from build123d import *

# Parameters (mm, degrees)
CROQUIS1_W              = 40
CROQUIS1_H              = 19
SALIENTE_EXTRUIR1_DEPTH = 36
SALIENTE_EXTRUIR2_DEPTH = 2.5
REDONDEO1_R             = 0.5
REDONDEO2_R             = 0.5
SALIENTE_EXTRUIR3_DEPTH = 2
SALIENTE_EXTRUIR4_DEPTH = 2
CROQUIS5_R              = 6.5
SALIENTE_EXTRUIR5_DEPTH = 1
CROQUIS6_R              = 5
SALIENTE_EXTRUIR6_DEPTH = 0.5
CROQUIS7_R              = 3
SALIENTE_EXTRUIR7_DEPTH = 5
SALIENTE_EXTRUIR8_START = -4
CROQUIS8_R              = 3
SALIENTE_EXTRUIR8_DEPTH = 4
CROQUIS9_R              = 2
CORTAR_EXTRUIR1_DEPTH   = 5
CHAFL_N1_SIZE           = 0.25
SALIENTE_EXTRUIR9_DEPTH = 1.75


with BuildPart() as part:
    # Croquis1 → Saliente-Extruir1 (new body)
    with BuildSketch(Plane(origin=(0, 0, 0), x_dir=(1, 0, 0), z_dir=(0, 1, 0))):
        with Locations((20, -9.5)):
            Rectangle(CROQUIS1_W, CROQUIS1_H)
    extrude(amount=SALIENTE_EXTRUIR1_DEPTH)

    # Croquis2 → Saliente-Extruir2 (add)
    with BuildSketch(Plane(origin=(0, 31, 0), x_dir=(-1, 0, 0), z_dir=(0, 1, 0))):
        with BuildLine():
            ThreePointArc((-46.515564437, 3.5), (-42.25, 4.5), (-46.515564437, 5.5))
            Line((-46.515564437, 5.5), (-47.5, 5.5))
            Line((-47.5, 5.5), (-47.5, 13.5))
            Line((-47.5, 13.5), (-46.515564437, 13.5))
            ThreePointArc((-46.515564437, 13.5), (-42.25, 14.5), (-46.515564437, 15.5))
            Line((-46.515564437, 15.5), (-47.5, 15.5))
            Line((-47.5, 15.5), (-47.5, 18.25))
            Line((-47.5, 18.25), (-40, 18.25))
            Line((-40, 18.25), (-40, 0.75))
            Line((-40, 0.75), (-47.5, 0.75))
            Line((-47.5, 0.75), (-47.5, 3.5))
            Line((-47.5, 3.5), (-46.515564437, 3.5))
        make_face()
        with BuildLine():
            Line((6.515564437, 13.5), (7.5, 13.5))
            Line((7.5, 13.5), (7.5, 5.5))
            Line((7.5, 5.5), (6.515564437, 5.5))
            ThreePointArc((6.515564437, 5.5), (2.25, 4.5), (6.515564437, 3.5))
            Line((6.515564437, 3.5), (7.5, 3.5))
            Line((7.5, 3.5), (7.5, 0.75))
            Line((7.5, 0.75), (0, 0.75))
            Line((0, 0.75), (0, 18.25))
            Line((0, 18.25), (7.5, 18.25))
            Line((7.5, 18.25), (7.5, 15.5))
            Line((7.5, 15.5), (6.515564437, 15.5))
            ThreePointArc((6.515564437, 15.5), (2.25, 14.5), (6.515564437, 13.5))
        make_face()
    extrude(amount=-SALIENTE_EXTRUIR2_DEPTH)

    # Redondeo1
    redondeo1_edges = [part.edges().sort_by_distance(p)[0] for p in [
        (0, 18, 0),
        (40, 18, 0),
        (40, 18, 19),
        (0, 18, 19),
    ]]
    fillet(redondeo1_edges, radius=REDONDEO1_R)

    # Redondeo2
    redondeo2_edges = [part.edges().sort_by_distance(p)[0] for p in [
        (0, 36, 9.5),
        (20, 36, 0),
        (20, 36, 19),
        (40, 36, 9.5),
        (39.853553391, 36, 18.853553391),
        (39.853553391, 36, 0.146446609),
        (0.146446609, 36, 18.853553391),
        (0.146446609, 36, 0.146446609),
    ]]
    fillet(redondeo2_edges, radius=REDONDEO2_R)

    # Croquis3 → Saliente-Extruir3 (add)
    with BuildSketch(Plane(origin=(0, 36, 0), x_dir=(1, 0, 0), z_dir=(0, 1, 0))):
        with BuildLine():
            Line((34.5, -18.25), (34.5, -0.75))
            Line((34.5, -0.75), (14.5, -0.75))
            Line((14.5, -0.75), (13.699662147, -0.75))
            ThreePointArc((13.699662147, -0.75), (17.918231823, -4.25103774), (19.5, -9.5))
            ThreePointArc((19.5, -9.5), (17.918231823, -14.74896226), (13.699662147, -18.25))
            Line((13.699662147, -18.25), (14.5, -18.25))
            Line((14.5, -18.25), (34.5, -18.25))
        make_face()
    extrude(amount=SALIENTE_EXTRUIR3_DEPTH)

    # Croquis4 → Saliente-Extruir4 (add, symmetric)
    with BuildSketch(Plane(origin=(0, 36, 0), x_dir=(1, 0, 0), z_dir=(0, 1, 0))):
        with BuildLine():
            ThreePointArc((19.5, -9.5), (17.918231823, -4.25103774), (13.699662147, -0.75))
            ThreePointArc((13.699662147, -0.75), (13.3728388, -0.618898805), (13.041381265, -0.5))
            Line((13.041381265, -0.5), (6.958618735, -0.5))
            ThreePointArc((6.958618735, -0.5), (0.5, -9.5), (6.958618735, -18.5))
            Line((6.958618735, -18.5), (13.041381265, -18.5))
            ThreePointArc((13.041381265, -18.5), (13.3728388, -18.381101195), (13.699662147, -18.25))
            ThreePointArc((13.699662147, -18.25), (17.918231823, -14.74896226), (19.5, -9.5))
        make_face()
        with BuildLine():
            ThreePointArc((6.958618735, -18.5), (10, -19), (13.041381265, -18.5))
            Line((13.041381265, -18.5), (6.958618735, -18.5))
        make_face()
        with BuildLine():
            Line((6.958618735, -0.5), (13.041381265, -0.5))
            ThreePointArc((13.041381265, -0.5), (10, 0), (6.958618735, -0.5))
        make_face()
    extrude(amount=SALIENTE_EXTRUIR4_DEPTH, both=True)

    # Croquis5 → Saliente-Extruir5 (add)
    with BuildSketch(Plane(origin=(0, 38, 0), x_dir=(1, 0, 0), z_dir=(0, 1, 0))):
        with Locations(Location((10, -9.5, 0), (0, 0, 270))):
            Circle(CROQUIS5_R)
    extrude(amount=SALIENTE_EXTRUIR5_DEPTH)

    # Croquis6 → Saliente-Extruir6 (add)
    with BuildSketch(Plane(origin=(0, 39, 0), x_dir=(1, 0, 0), z_dir=(0, 1, 0))):
        with Locations(Location((10, -9.5, 0), (0, 0, 270))):
            Circle(CROQUIS6_R)
    extrude(amount=SALIENTE_EXTRUIR6_DEPTH)

    # Croquis7 → Saliente-Extruir7 (add)
    with BuildSketch(Plane(origin=(0, 39.5, 0), x_dir=(1, 0, 0), z_dir=(0, 1, 0))):
        with Locations(Location((10, -9.5, 0), (0, 0, 270))):
            Circle(CROQUIS7_R)
    extrude(amount=SALIENTE_EXTRUIR7_DEPTH)

    # Croquis8 → Saliente-Extruir8 (add)
    with BuildSketch(Plane(origin=(0, 44.5, 0), x_dir=(1, 0, 0), z_dir=(0, 1, 0)).offset(SALIENTE_EXTRUIR8_START)):
        with Locations(Location((10, -9.5, 0), (0, 0, 270))):
            Circle(CROQUIS8_R)
        with BuildLine():
            ThreePointArc((8.5, -6.901923789), (8.11283957, -7.040604645), (7.878679656, -7.378679656))
            ThreePointArc((7.878679656, -7.378679656), (8.173715713, -7.119939979), (8.5, -6.901923789))
        make_face()
        with BuildLine():
            ThreePointArc((9.223542865, -6.602222521), (8.81368136, -6.635973449), (8.5, -6.901923789))
            ThreePointArc((8.5, -6.901923789), (8.851949703, -6.728361402), (9.223542865, -6.602222521))
        make_face()
        with BuildLine():
            ThreePointArc((10, -6.5), (9.595368804, -6.42652093), (9.223542865, -6.602222521))
            ThreePointArc((9.223542865, -6.602222521), (9.608421423, -6.525665416), (10, -6.5))
        make_face()
        with BuildLine():
            ThreePointArc((10.776457135, -6.602222521), (10.404631196, -6.42652093), (10, -6.5))
            ThreePointArc((10, -6.5), (10.391578577, -6.525665416), (10.776457135, -6.602222521))
        make_face()
        with BuildLine():
            ThreePointArc((11.5, -6.901923789), (11.18631864, -6.635973449), (10.776457135, -6.602222521))
            ThreePointArc((10.776457135, -6.602222521), (11.148050297, -6.728361402), (11.5, -6.901923789))
        make_face()
        with BuildLine():
            ThreePointArc((12.121320344, -7.378679656), (11.88716043, -7.040604645), (11.5, -6.901923789))
            ThreePointArc((11.5, -6.901923789), (11.826284287, -7.119939979), (12.121320344, -7.378679656))
        make_face()
        with BuildLine():
            ThreePointArc((12.598076211, -8), (12.771638598, -8.351949703), (12.897777479, -8.723542865))
            ThreePointArc((12.897777479, -8.723542865), (12.864026551, -8.31368136), (12.598076211, -8))
        make_face()
        with BuildLine():
            ThreePointArc((12.897777479, -8.723542865), (12.974334584, -9.108421423), (13, -9.5))
            ThreePointArc((13, -9.5), (13.07347907, -9.095368804), (12.897777479, -8.723542865))
        make_face()
        with BuildLine():
            ThreePointArc((12.121320344, -7.378679656), (12.380060021, -7.673715713), (12.598076211, -8))
            ThreePointArc((12.598076211, -8), (12.459395355, -7.61283957), (12.121320344, -7.378679656))
        make_face()
        with BuildLine():
            ThreePointArc((7.878679656, -7.378679656), (7.540604645, -7.61283957), (7.401923789, -8))
            ThreePointArc((7.401923789, -8), (7.619939979, -7.673715713), (7.878679656, -7.378679656))
        make_face()
        with BuildLine():
            ThreePointArc((7.401923789, -11), (7.440963384, -11.204433973), (7.540604645, -11.38716043))
            ThreePointArc((7.540604645, -11.38716043), (7.691315793, -11.530699585), (7.878679656, -11.621320344))
            ThreePointArc((7.878679656, -11.621320344), (7.619939979, -11.326284287), (7.401923789, -11))
        make_face()
        with BuildLine():
            ThreePointArc((7.102222521, -10.276457135), (7.135973449, -10.68631864), (7.401923789, -11))
            ThreePointArc((7.401923789, -11), (7.228361402, -10.648050297), (7.102222521, -10.276457135))
        make_face()
        with BuildLine():
            ThreePointArc((7, -9.5), (6.92652093, -9.904631196), (7.102222521, -10.276457135))
            ThreePointArc((7.102222521, -10.276457135), (7.025665416, -9.891578577), (7, -9.5))
        make_face()
        with BuildLine():
            ThreePointArc((7.102222521, -8.723542865), (6.92652093, -9.095368804), (7, -9.5))
            ThreePointArc((7, -9.5), (7.025665416, -9.108421423), (7.102222521, -8.723542865))
        make_face()
        with BuildLine():
            ThreePointArc((7.401923789, -8), (7.135973449, -8.31368136), (7.102222521, -8.723542865))
            ThreePointArc((7.102222521, -8.723542865), (7.228361402, -8.351949703), (7.401923789, -8))
        make_face()
        with BuildLine():
            ThreePointArc((7.878679656, -11.621320344), (7.969300415, -11.808684207), (8.11283957, -11.959395355))
            ThreePointArc((8.11283957, -11.959395355), (8.295566027, -12.059036616), (8.5, -12.098076211))
            ThreePointArc((8.5, -12.098076211), (8.173715713, -11.880060021), (7.878679656, -11.621320344))
        make_face()
        with BuildLine():
            ThreePointArc((9.223542865, -12.397777479), (8.851949703, -12.271638598), (8.5, -12.098076211))
            ThreePointArc((8.5, -12.098076211), (8.81368136, -12.364026551), (9.223542865, -12.397777479))
        make_face()
        with BuildLine():
            ThreePointArc((10, -12.5), (9.608421423, -12.474334584), (9.223542865, -12.397777479))
            ThreePointArc((9.223542865, -12.397777479), (9.595368804, -12.57347907), (10, -12.5))
        make_face()
        with BuildLine():
            ThreePointArc((10.776457135, -12.397777479), (10.391578577, -12.474334584), (10, -12.5))
            ThreePointArc((10, -12.5), (10.404631196, -12.57347907), (10.776457135, -12.397777479))
        make_face()
        with BuildLine():
            ThreePointArc((11.5, -12.098076211), (11.148050297, -12.271638598), (10.776457135, -12.397777479))
            ThreePointArc((10.776457135, -12.397777479), (11.18631864, -12.364026551), (11.5, -12.098076211))
        make_face()
        with BuildLine():
            ThreePointArc((12.121320344, -11.621320344), (11.826284287, -11.880060021), (11.5, -12.098076211))
            ThreePointArc((11.5, -12.098076211), (11.88716043, -11.959395355), (12.121320344, -11.621320344))
        make_face()
        with BuildLine():
            ThreePointArc((12.598076211, -11), (12.380060021, -11.326284287), (12.121320344, -11.621320344))
            ThreePointArc((12.121320344, -11.621320344), (12.459395355, -11.38716043), (12.598076211, -11))
        make_face()
        with BuildLine():
            ThreePointArc((12.897777479, -10.276457135), (12.771638598, -10.648050297), (12.598076211, -11))
            ThreePointArc((12.598076211, -11), (12.864026551, -10.68631864), (12.897777479, -10.276457135))
        make_face()
        with BuildLine():
            ThreePointArc((13, -9.5), (12.974334584, -9.891578577), (12.897777479, -10.276457135))
            ThreePointArc((12.897777479, -10.276457135), (13.07347907, -9.904631196), (13, -9.5))
        make_face()
    extrude(amount=SALIENTE_EXTRUIR8_DEPTH)

    # Croquis9 → Cortar-Extruir1 (cut)
    with BuildSketch(Plane(origin=(0, 44.5, 0), x_dir=(1, 0, 0), z_dir=(0, 1, 0))):
        with Locations(Location((10, -9.5, 0), (0, 0, 270))):
            Circle(CROQUIS9_R)
    extrude(amount=-CORTAR_EXTRUIR1_DEPTH, mode=Mode.SUBTRACT)

    # Chaflán1
    chafl_n1_edges = [part.edges().sort_by_distance(p)[0] for p in [
        (10, 44.5, 7.5),
    ]]
    chamfer(chafl_n1_edges, length=CHAFL_N1_SIZE)

    # Croquis10 → Saliente-Extruir9 (add)
    with BuildSketch(Plane(origin=(0, 36, 0), x_dir=(1, 0, 0), z_dir=(0, 1, 0))):
        with BuildLine():
            ThreePointArc((34.5, -14), (36, -9.5), (34.5, -5))
            Line((34.5, -5), (34.5, -14))
        make_face()
    extrude(amount=SALIENTE_EXTRUIR9_DEPTH)


solid = part.part
For this review, take the finished solid that the model builds, in its own axes (mm). A direction names the side the tool comes from. Give positions to 0.01 mm unless a question says otherwise; leave off trailing zeros. Loops run counter-clockwise (first coordinate to the right, second up) from the corner with the lowest first, then second, coordinate; pieces in that order, holes last. Notation, with made-up numbers: M -20.75,15.5 L 29.25,15.5 A15 cw 29.25,26.5 Z; hole C 4.5,-14.5 d11. An arc over 180 degrees is marked long. Put each result on its own line as item: value. Start each with the question number.
(1) Machinability: for faces 5 (the flat face through (10, 39.5, 9)), 6 (the flat face through (-3, 31, 10)), 7 (the flat face through (44, 30, 0.75)), which of the approach directions +Z, -Z, +X, -X, +Y, -Y give a long, thin tool a straight path to every point of the face, cutting with its end or side? Answer none if there is none.
(2) Add section C-C, the plane x = 33.5. Write out the cut boundary in (y, z), then the cut area to 3 significant figures.
(3) The part is to be moulded in two halves that separate along Z. For faces 1 (the flat face through (47.5, 30, 9)), 2 (the cylindrical face through (42.25, 29.77, 4.42)), 3 (the flat face through (44, 30, 18.25)), 4 (the flat face through (-4, 30, 0.75)), say which applies: +Z half, -Z half, draft (parallel to the pull), parting line (faces both ways), or undercut.
(4) Wall thickness on L1, parallel to Z at x = -4.5, y = 29.5; L2, parallel to X at y = 42.4, z = 9.5; L3, parallel to Y at x = 29, z = 16: over which ranges is each line inside the solid? List them lowest first.
(5) For pin 1 (3 mm diameter, centred on x = 29, z = 4, fed in from -Y); pin 2 (1.5 mm diameter, centred on x = 41, z = 16, fed in from -Y); pin 3 (2.5 mm diameter, centred on x = 44.5, z = 4.5, fed in from +Y); pin 4 (2 mm diameter, centred on x = 36, z = 12.5, fed in from +Y), all flat-tipped, find the tip position at first contact; note any pin that passes through.
(6) Add section A-A, the plane x = -4.5. Write out the cut boundary in (y, z).
Result:
1. face 5: +Y
1. face 6: +Z, -Z, -X, +Y
1. face 7: -Z, +X, +Y, -Y
2. outline: M 0,0 L 35.5,0 A0.5 ccw 36,0.5 L 36,0.75 L 38,0.75 L 38,18.25 L 36,18.25 L 36,18.5 A0.5 ccw 35.5,19 L 0,19 Z
2. area: 719 mm^2
3. face 1: draft
3. face 2: undercut
3. face 3: +Z half
3. face 4: -Z half
4. L1: z = 0.75 to 2.25, 6.75 to 12.25, 16.75 to 18.25
4. L2: x = 7 to 8, 12 to 13
4. L3: y = 0 to 38
5. pin 1: stops at y = 0
5. pin 2: stops at y = 28.5
5. pin 3: passes through
5. pin 4: stops at y = 37.75
6. outline: M 28.5,0.75 L 31,0.75 L 31,2.25 L 28.5,2.25 Z; M 28.5,6.75 L 31,6.75 L 31,12.25 L 28.5,12.25 Z; M 28.5,16.75 L 31,16.75 L 31,18.25 L 28.5,18.25 Z
